Part model, mm, in its own coordinate system. Round coordinates to 2 decimals unless told otherwise and drop trailing zeros. Write each loop counter-clockwise with the first axis right and the second up, starting at its lowest first coordinate (ties: lowest second). Pieces come first, ordered by that corner, then holes. Notation, with made-up numbers: M 1,88.5 L 36,88.5 A20 ccw 36,105.5 Z; hole C 32.25,48.25 d1. An arc over 180 degrees is marked long. Answer as a JSON object with one key per item and string values. Group by question number.
1. Band-saw the part on B-B, the plane z = -585. Write the cut outline in (x, y), plus the area to 3 significant figures.
2. Band-saw the part on A-A, the plane x = 0. Write the cut outline in (y, z).
3. Drop flat-ended pins along their axis: pin 1 (6 mm diameter, centred on x = 5.5, z = -1440, fed in from -Y); pin 2 (3 mm diameter, centred on x = 8.5, y = 9, fed in from +Z); pin 3 (12 mm diameter, centred on x = 1, y = -48.5, fed in from +Z). Give the stop position or say it passes through.
4. Drill centre lines: line 1 (Y direction, x = 1.75, z = -842.5); line 2 (Y direction, x = 2.5, z = -1294.5); line 3 (X direction, y = 105, z = -698.5). Where is each one in solid material? Low to high. Write a range as from..to.
from build123d import *

# Parameters (mm, degrees)
SKETCH2_R   = 10.65
SKETCH2_R_2 = 6.92


with BuildPart() as part:
    # Sweep1: sweep along a path in Sketch1
    with BuildLine(Plane(origin=(0, 0, 0), x_dir=(0, 0, -1), z_dir=(1, 0, 0))) as sweep1_path:
        Line((0, 105), (2325, 105))
        ThreePointArc((2325, 105), (2430, 0), (2325, -105))
        Line((2325, -105), (0, -105))
    # Sketch2 → Sweep1 (sweep)
    with BuildSketch(Plane.XY):
        with Locations((0, 105)):
            Circle(SKETCH2_R)
        with Locations((0, 105)):
            Circle(SKETCH2_R_2, mode=Mode.SUBTRACT)
    sweep(path=sweep1_path.line)


solid = part.part
Worked answers:
{
 "1": {"outline": "C 0,-105 d21.3; C 0,105 d21.3; hole C 0,-105 d13.84; hole C 0,105 d13.84", "area": "412 mm^2"},
 "2": {"outline": "M -115.65,-2325 A115.65 ccw 115.65,-2325 L 115.65,0 L 111.92,0 L 111.92,-2325 A111.92 cw -111.92,-2325 L -111.92,0 L -115.65,0 Z; M -98.08,-2325 A98.08 ccw 98.08,-2325 L 98.08,0 L 94.35,0 L 94.35,-2325 A94.35 cw -94.35,-2325 L -94.35,0 L -98.08,0 Z"},
 "3": {"pin 1": "stops at y = -115.35", "pin 2": "stops at z = -2421.55", "pin 3": "stops at z = -2402.05"},
 "4": {"line 1": "y = -115.51..-111.7, -98.3..-94.49, 94.49..98.3, 111.7..115.51", "line 2": "y = -115.35..-111.45, -98.55..-94.65, 94.65..98.55, 111.45..115.35", "line 3": "x = -10.65..-6.92, 6.92..10.65"}
}
